Read the model definition and answer for the solid it produces. Units are mm, in the model's axes. A direction names the side the tool comes from. Round coordinates to 2 decimals unless told otherwise and drop trailing zeros. Loops run counter-clockwise (first coordinate to the right, second up) from the corner with the lowest first, then second, coordinate; pieces in that order, holes last. Notation, with made-up numbers: (15.5, -36.75) - (44.5, -36.75) arc R35 ccw to (44.5, -3.75) - close; hole circle Ø10 at (-15, -4.75). An arc over 180 degrees is marked (long way). Answer as CSV lines item,"result".
```python
from build123d import *

# Parameters (mm, degrees)
EXTRUDE_1_DEPTH     = 20
SKETCH_2_R          = 4
EXTRUDE_2_DEPTH     = 8
SKETCH_3_R          = 2.5
CUT_EXTRUDE_1_DEPTH = 20


with BuildPart() as part:
    # 草图1 → 凸台-拉伸1 (new body)
    with BuildSketch(Plane.XY):
        with BuildLine():
            Line((3.195386911, 4.038125731), (2.251763738, 3.305988516))
            ThreePointArc((2.251763738, 3.305988516), (-3.160315011, -2.452021418), (3.761777443, 1.359790599))
            Line((3.761777443, 1.359790599), (4.705400616, 2.091927813))
            Line((4.705400616, 2.091927813), (3.195386911, 4.038125731))
        make_face()
    extrude(amount=EXTRUDE_1_DEPTH)

    # 草图2 → 凸台-拉伸2 (add)
    with BuildSketch(Plane.XY.offset(20)):
        with Locations(Location((0, 0, 0), (0, 0, 55.740572038))):
            Circle(SKETCH_2_R)
    extrude(amount=EXTRUDE_2_DEPTH)

    # 草图3 → 切除-拉伸1 (cut)
    with BuildSketch(Plane.XY.offset(28)):
        Circle(SKETCH_3_R)
    extrude(amount=-CUT_EXTRUDE_1_DEPTH, mode=Mode.SUBTRACT)


solid = part.part
```
1) Find the intervals of material crossed by line 1 (Y direction, x = 0, z = 13.25); line 2 (X direction, y = -0.75, z = 25); line 3 (Z direction, x = 1.25, y = -1.5), in increasing order.
Entries:
line 1,"y = -4 to -2.5, 2.5 to 4"
line 2,"x = -3.93 to -2.38, 2.38 to 3.93"
line 3,"z = 0 to 8"
2) A tool of negligible diameter and unlimited length cuts with its end or side. For faces 4 (the face through (2.73, 3.677, 9.86)), 5 (the face through (0, 0, 8)), 6 (the face through (2, -2, 28)), from which of +Z, -Z, +X, -X, +Y, -Y can it reach the whole face along a straight path? Write none if from no direction.
Entries:
face 4,"+Z, -Z, +Y"
face 5,"+Z"
face 6,"+Z, +X, -X, +Y, -Y"
3) Each of these flat-tipped pins is pushed along its axis until it touches: P1, Ø1.5, axis at x = 2.5, z = 7.5, coming from the -Y side; P2, Ø2, axis at x = 1, z = 22.5, coming from the +Y side; P3, Ø2, axis at y = -1, z = 21, coming from the +X side. Where does it stop, or does it pass through?
Entries:
P1,"stops at y = -3.6"
P2,"stops at y = 4"
P3,"stops at x = 4"
4) A cutting plane is placed at B-B, the plane x = 0. Determine the outline of the cut face in (y, z), plus the area to 3 significant figures.
Entries:
outline,"(-4, 0) - (4, 0) - (4, 28) - (2.5, 28) - (2.5, 8) - (-2.5, 8) - (-2.5, 28) - (-4, 28) - close"
area,"124 mm^2"
5) The mould has two halves that part along Y. Classify faces 1 (the face through (4, 3, 10)), 2 (the face through (4.2, 1.7, 9.9)), 3 (the face through (3, 3, 20)): pulls with the +Y half, pulls with the -Y half, needs draft (parallel to the pull), parting line crosses it, or undercut.
Entries:
face 1,"pulls with the +Y half"
face 2,"undercut"
face 3,"needs draft"
6) A cutting plane is placed at D-D, the plane z = 5.75. Determine the outline of the cut face in (x, y).
Entries:
outline,"(2.25, 3.31) arc R4 ccw (long way) to (3.76, 1.36) - (4.71, 2.09) - (3.2, 4.04) - close"
7) A cutting plane is placed at A-A, the plane z = 12.5. Determine the outline of the cut face in (x, y), plus the area to 3 significant figures.
Entries:
outline,"(2.25, 3.31) arc R4 ccw (long way) to (3.76, 1.36) - (4.71, 2.09) - (3.2, 4.04) - close; hole circle Ø5 at (0, 0)"
area,"33.3 mm^2"
